```python
from build123d import *

# Parameters (mm, degrees)
SKETCH_1_W          = 145
SKETCH_1_H          = 80
EXTRUDE_1_DEPTH     = 2
FILLET_1_R          = 20
CUT_EXTRUDE_1_DEPTH = 2
EXTRUDE_2_DEPTH     = 2
EXTRUDE_4_DEPTH     = 7.5
EXTRUDE_5_DEPTH     = 30
FILLET_2_R          = 0.5
EXTRUDE_6_DEPTH     = 4.7
EXTRUDE_START       = -1.5
EXTRUDE_9_DEPTH     = 1.5
CHAMFER_2_SIZE      = 3
SKETCH_11_R         = 1
CUT_EXTRUDE_2_DEPTH = 149.399637803
CHAMFER_3_SIZE      = 0.5
EXTRUDE_10_DEPTH    = 60


with BuildPart() as part:
    # Эскиз1 → Бобышка-Вытянуть1 (new body)
    with BuildSketch(Plane(origin=(0, 0, 0), x_dir=(1, 0, 0), z_dir=(0, 1, 0))):
        Rectangle(SKETCH_1_W, SKETCH_1_H)
    extrude(amount=EXTRUDE_1_DEPTH)

    # Скругление1
    fillet_1_edges = [part.edges().sort_by_distance(p)[0] for p in [
        (72.5, 1, 40),
        (-72.5, 1, 40),
    ]]
    fillet(fillet_1_edges, radius=FILLET_1_R)

    # Эскиз2 → Вырез-Вытянуть1 (cut)
    with BuildSketch(Plane(origin=(0, 2, 0), x_dir=(1, 0, 0), z_dir=(0, 1, 0))):
        with BuildLine():
            Line((-63.5, 31), (-63.5, -20))
            ThreePointArc((-63.5, -20), (-60.278174593, -27.778174593), (-52.5, -31))
            Line((-52.5, -31), (52.5, -31))
            ThreePointArc((52.5, -31), (60.278174593, -27.778174593), (63.5, -20))
            Line((63.5, -20), (63.5, 31))
            Line((63.5, 31), (-63.5, 31))
        make_face()
    extrude(amount=-CUT_EXTRUDE_1_DEPTH, mode=Mode.SUBTRACT)

    # Эскиз3 → Бобышка-Вытянуть2 (add)
    with BuildSketch(Plane.XZ):
        with BuildLine():
            Line((70.25, -37.75), (70.25, 20))
            ThreePointArc((70.25, 20), (65.051145366, 32.551145366), (52.5, 37.75))
            Line((52.5, 37.75), (-52.5, 37.75))
            ThreePointArc((-52.5, 37.75), (-65.051145366, 32.551145366), (-70.25, 20))
            Line((-70.25, 20), (-70.25, -37.75))
            Line((-70.25, -37.75), (70.25, -37.75))
        make_face()
        with BuildLine():
            Line((-63.5, -31), (-63.5, 20))
            ThreePointArc((-63.5, 20), (-60.278174593, 27.778174593), (-52.5, 31))
            Line((-52.5, 31), (52.5, 31))
            ThreePointArc((52.5, 31), (60.278174593, 27.778174593), (63.5, 20))
            Line((63.5, 20), (63.5, -31))
            Line((63.5, -31), (-63.5, -31))
        make_face(mode=Mode.SUBTRACT)
    extrude(amount=EXTRUDE_2_DEPTH)

    # Эскиз5 → Бобышка-Вытянуть4 (add, symmetric)
    with BuildSketch(Plane(origin=(0, 0, 0), x_dir=(0, 0, -1), z_dir=(1, 0, 0))):
        Polygon((37.75, -2), (31, -2), (31, -6.7), (37.75, -6.7), (39.45, -5), (37.75, -3.3), align=None)
        Polygon((-31, -2), (-31, -6.7), (-37.75, -6.7), (-39.45, -5), (-37.75, -3.3), (-37.75, -2), align=None)
    extrude(amount=EXTRUDE_4_DEPTH, both=True)

    # Эскиз6 → Бобышка-Вытянуть5 (add, symmetric)
    with BuildSketch(Plane(origin=(0, 0, 0), x_dir=(0, 0, -1), z_dir=(1, 0, 0))):
        Polygon((-39.45, -5), (-37.75, -6.7), (-31, -6.7), (-31, -2), (-37.75, -2), (-37.75, -3.3), align=None)
    extrude(amount=EXTRUDE_5_DEPTH, both=True)

    # Скругление2
    fillet_2_edges = [part.edges().sort_by_distance(p)[0] for p in [
        (0, -5, 39.45),
        (0, -5, -39.45),
    ]]
    fillet(fillet_2_edges, radius=FILLET_2_R)

    # Эскиз7 → Бобышка-Вытянуть6 (add)
    with BuildSketch(Plane.XZ.offset(2)):
        with BuildLine():
            Line((-52.5, 31), (-30, 31))
            Line((-30, 31), (-30, 37.75))
            Line((-30, 37.75), (-52.5, 37.75))
            ThreePointArc((-52.5, 37.75), (-65.051145366, 32.551145366), (-70.25, 20))
            Line((-70.25, 20), (-70.25, -37.75))
            Line((-70.25, -37.75), (-7.5, -37.75))
            Line((-7.5, -37.75), (-7.5, -31))
            Line((-7.5, -31), (-63.5, -31))
            Line((-63.5, -31), (-63.5, 20))
            ThreePointArc((-63.5, 20), (-60.278174593, 27.778174593), (-52.5, 31))
        make_face()
        with BuildLine():
            Line((30, 31), (52.5, 31))
            ThreePointArc((52.5, 31), (60.278174593, 27.778174593), (63.5, 20))
            Line((63.5, 20), (63.5, -31))
            Line((63.5, -31), (7.5, -31))
            Line((7.5, -31), (7.5, -37.75))
            Line((7.5, -37.75), (70.25, -37.75))
            Line((70.25, -37.75), (70.25, 20))
            ThreePointArc((70.25, 20), (65.051145366, 32.551145366), (52.5, 37.75))
            Line((52.5, 37.75), (30, 37.75))
            Line((30, 37.75), (30, 31))
        make_face()
    extrude(amount=EXTRUDE_6_DEPTH)

    # Эскиз10 → Бобышка-Вытянуть9 (add)
    with BuildSketch(Plane.XZ.offset(6.7).offset(EXTRUDE_START)):
        with BuildLine():
            Line((-63.5, 20), (-63.5, -31))
            Line((-63.5, -31), (63.5, -31))
            Line((63.5, -31), (63.5, 20))
            ThreePointArc((63.5, 20), (60.278174593, 27.778174593), (52.5, 31))
            Line((52.5, 31), (-52.5, 31))
            ThreePointArc((-52.5, 31), (-60.278174593, 27.778174593), (-63.5, 20))
        make_face()
        with BuildLine():
            Line((60.5, -28), (60.5, 20))
            ThreePointArc((60.5, 20), (58.156854249, 25.656854249), (52.5, 28))
            Line((52.5, 28), (-52.5, 28))
            ThreePointArc((-52.5, 28), (-58.156854249, 25.656854249), (-60.5, 20))
            Line((-60.5, 20), (-60.5, -28))
            Line((-60.5, -28), (60.5, -28))
        make_face(mode=Mode.SUBTRACT)
    extrude(amount=EXTRUDE_9_DEPTH)

    # Фаска2
    chamfer_2_edges = [part.edges().sort_by_distance(p)[0] for p in [
        (-60.278174593, -5.2, 27.778174593),
        (0, -5.2, 31),
        (60.278174593, -5.2, 27.778174593),
        (63.5, -5.2, -5.5),
        (0, -5.2, -31),
        (-63.5, -5.2, -5.5),
    ]]
    chamfer(chamfer_2_edges, length=CHAMFER_2_SIZE - 0.0001)  # a hair under: the kernel refuses the full size

    # Эскиз11 → Вырез-Вытянуть2 (cut, through all)
    with BuildSketch(Plane(origin=(70.25, 0, 0), x_dir=(0, 0, -1), z_dir=(1, 0, 0))):
        with Locations((28, -1)):
            Circle(SKETCH_11_R)
    extrude(amount=-CUT_EXTRUDE_2_DEPTH, mode=Mode.SUBTRACT)

    # Фаска3
    chamfer_3_edges = [part.edges().sort_by_distance(p)[0] for p in [
        (0, 2, -31),
        (-63.5, 2, -5.5),
        (-60.278174593, 2, 27.778174593),
        (0, 2, 31),
        (60.278174593, 2, 27.778174593),
        (63.5, 2, -5.5),
    ]]
    chamfer(chamfer_3_edges, length=CHAMFER_3_SIZE)

    # Эскиз12 → Бобышка-Вытянуть10 (add, symmetric)
    with BuildSketch(Plane(origin=(0, 0, 0), x_dir=(0, 0, -1), z_dir=(1, 0, 0))):
        with BuildLine():
            Line((39.096446609, -4.646446609), (37.75, -3.3))
            Line((37.75, -3.3), (37.75, -6.7))
            Line((37.75, -6.7), (39.096446609, -5.353553391))
            ThreePointArc((39.096446609, -5.353553391), (39.242893219, -5), (39.096446609, -4.646446609))
        make_face()
    extrude(amount=EXTRUDE_10_DEPTH, both=True)


solid = part.part
```
Here's how the part is built. I have some questions about the finished solid (model axes, mm). A direction names the side the tool comes from. Coordinates: 2 decimals unless noted, no trailing zeros. One line per item, written item: value.
1) We'd pull the mould along Y, two halves only. Please class faces 6 (the conical face through (-60.465, 1.642, 27.792)), 7 (the flat face through (-1, -2, -37.75)), 8 (the flat face through (-63.5, 0, -6)): pulls with the +Y half, pulls with the -Y half, needs draft (parallel to the pull), parting line crosses it, or undercut.
Model answer:
face 6: pulls with the +Y half
face 7: undercut
face 8: needs draft
2) I need wall thicknesses on line 1 along Z through (x, y) = (-26.5, -0.5); line 2 along Y through (x, z) = (68, -28); line 3 along X through (y, z) = (-2, 16.5). Which ranges of each line are inside material? Lowest first, please.
Model answer:
line 1: z = -37.75 to -31, 31 to 37.75
line 2: y = -6.7 to -2, 0 to 2
line 3: x = -70.25 to -63.5, 63.5 to 70.25
3) I'm going to push flat-ended pins straight in: P1, Ø1.2, axis at y = -6, z = -12.5, coming from the +X side; P2, Ø1.2, axis at y = -5, z = -39, coming from the +X side; P3, Ø1.6, axis at y = -1, z = -28, coming from the +X side; P4, Ø3.5, axis at x = 4.5, y = -3.5, coming from the +Z side. Where does each tip first touch, or does it pass through?
Model answer:
P1: stops at x = 70.25
P2: stops at x = 60
P3: passes through
P4: stops at z = 39.24
4) On a 3-axis mill with a long thin cutter (end or side, diameter ignored), from which of +Z, -Z, +X, -X, +Y, -Y can I reach the whole of each face in a straight line? I mean faces 1 (the flat face through (1, -3, 37.75)), 2 (the flat face through (70.25, -3, -9)), 3 (the cylindrical face through (-58.094, -5.94, 25.719)), 4 (the cylindrical face through (65.2, -3.3, 32.4)), 5 (the conical face through (60.292, 1.642, 27.965)). Say none if no direction works.
Model answer:
face 1: +Z
face 2: +Z, -Z, +X, -Y
face 3: +Y, -Y
face 4: +Z, +X, -Y
face 5: +Y
